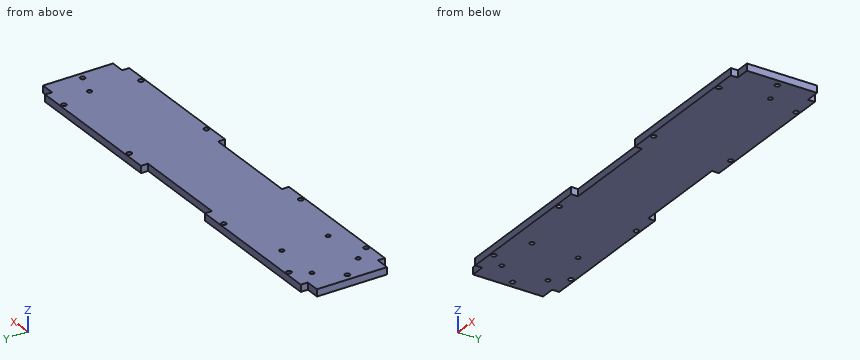
from build123d import *

# Parameters (mm, degrees)
SKETCH1_W           = 105
SKETCH1_H           = 5
SKETCH1_W_2         = 10
SKETCH1_H_2         = 50
BOSS_EXTRUDE1_DEPTH = 5
SKETCH2_R           = 1.75
CUT_EXTRUDE1_DEPTH  = 5
SKETCH3_R           = 1.75
CUT_EXTRUDE2_DEPTH  = 10
SKETCH5_R           = 1.575
CUT_EXTRUDE4_DEPTH  = 160.843673631


with BuildPart() as part:
    # Sketch1 → Boss-Extrude1 (new body)
    with BuildSketch(Plane.XY):
        Polygon((-35, 0), (0, 0), (0, 50), (-35, 50), (-140, 50), (-140, 0), align=None)
        Polygon((0, 50), (0, 0), (35, 0), (140, 0), (140, 50), (35, 50), align=None)
        with Locations((-87.5, -2.5)):
            Rectangle(SKETCH1_W, SKETCH1_H)
        with Locations((87.5, -2.5)):
            Rectangle(SKETCH1_W, SKETCH1_H)
        with Locations((-87.5, 52.5)):
            Rectangle(SKETCH1_W, SKETCH1_H)
        with Locations((87.5, 52.5)):
            Rectangle(SKETCH1_W, SKETCH1_H)
        with Locations((-145, 25)):
            Rectangle(SKETCH1_W_2, SKETCH1_H_2)
        with Locations((145, 25)):
            Rectangle(SKETCH1_W_2, SKETCH1_H_2)
    extrude(amount=BOSS_EXTRUDE1_DEPTH)

    # Sketch2 → Cut-Extrude1 (cut)
    with BuildSketch(Plane.XY.offset(5)):
        with Locations((-123.25, -2.5)):
            Circle(SKETCH2_R)
        with Locations(Location((-51.75, -2.5, 0), (0, 0, 180))):
            Circle(SKETCH2_R)
        with Locations((51.75, -2.5)):
            Circle(SKETCH2_R)
        with Locations(Location((123.25, -2.5, 0), (0, 0, 180))):
            Circle(SKETCH2_R)
        with Locations((123.25, 52.5)):
            Circle(SKETCH2_R)
        with Locations(Location((51.75, 52.5, 0), (0, 0, 180))):
            Circle(SKETCH2_R)
        with Locations((-51.75, 52.5)):
            Circle(SKETCH2_R)
        with Locations(Location((-123.25, 52.5, 0), (0, 0, 180))):
            Circle(SKETCH2_R)
    extrude(amount=-CUT_EXTRUDE1_DEPTH, mode=Mode.SUBTRACT)

    # Sketch3 → Cut-Extrude2 (cut)
    with BuildSketch(Plane.XY.offset(5)):
        with Locations((-145, 25)):
            Circle(SKETCH3_R)
        with Locations((145, 25)):
            Circle(SKETCH3_R)
    extrude(amount=-CUT_EXTRUDE2_DEPTH, mode=Mode.SUBTRACT)

    # Sketch5 → Cut-Extrude4 (cut, through all)
    with BuildSketch(Plane.XY.offset(5)):
        with Locations((-131.5, 41.5)):
            Circle(SKETCH5_R)
        with Locations(Location((-98.5, 41.5, 0), (0, 0, 180))):
            Circle(SKETCH5_R)
        with Locations((-98.5, 8.5)):
            Circle(SKETCH5_R)
        with Locations(Location((-131.5, 8.5, 0), (0, 0, 180))):
            Circle(SKETCH5_R)
        with Locations((128.87, 30.5)):
            Circle(SKETCH5_R)
    extrude(amount=-CUT_EXTRUDE4_DEPTH, mode=Mode.SUBTRACT)


solid = part.part
Input: part model. Units: mm. Frame: model coordinates. Give positions to 0.01 mm unless a question says otherwise; leave off trailing zeros. Order: outer loops, then holes, each group sorted by start corner. A loop starts at its lowest first (then second) coordinate and runs counter-clockwise, first axis right, second up.
Q1. Contact query for flat-ended pins moving along their axis: pin 1 Ø3 at (x, y) = (123.25, -2.5) entering from +Z; pin 2 Ø1.5 at (x, z) = (-145, 2.5) entering from +Y; pin 3 Ø1.5 at (y, z) = (51.5, 3.5) entering from +X. Output: stop coordinate, or through.
Checked values:
pin 1: passes through
pin 2: stops at y = 50
pin 3: stops at x = 140
Q2. Section A-A on z = 3.65. State how many separate pieces and enclosed holes the cut face has, and give its area (3 significant figures).
Checked values:
separate pieces: 1
enclosed holes: 15
area: 17,000 mm2
Q3. Ray query, probe 1 along Y at (x, z) = (-131.5, 1.4) (3 decimals); probe 2 along X at (y, z) = (51, 3.5); probe 3 along Y at (x, z) = (-131, 1). Return the intervals inside material, ascending.
Checked values:
probe 1: y = -5 to 6.925, 10.075 to 39.925, 43.075 to 55
probe 2: x = -140 to -124.15, -122.35 to -52.65, -50.85 to -35, 35 to 50.85, 52.65 to 122.35, 124.15 to 140
probe 3: y = -5 to 7.01, 9.99 to 40.01, 42.99 to 55
Q4. Section B-B on x = 28. Output: boundary loops of the cut face in (y, z).
Checked values:
outline: (0, 0) - (50, 0) - (50, 5) - (0, 5) - close
